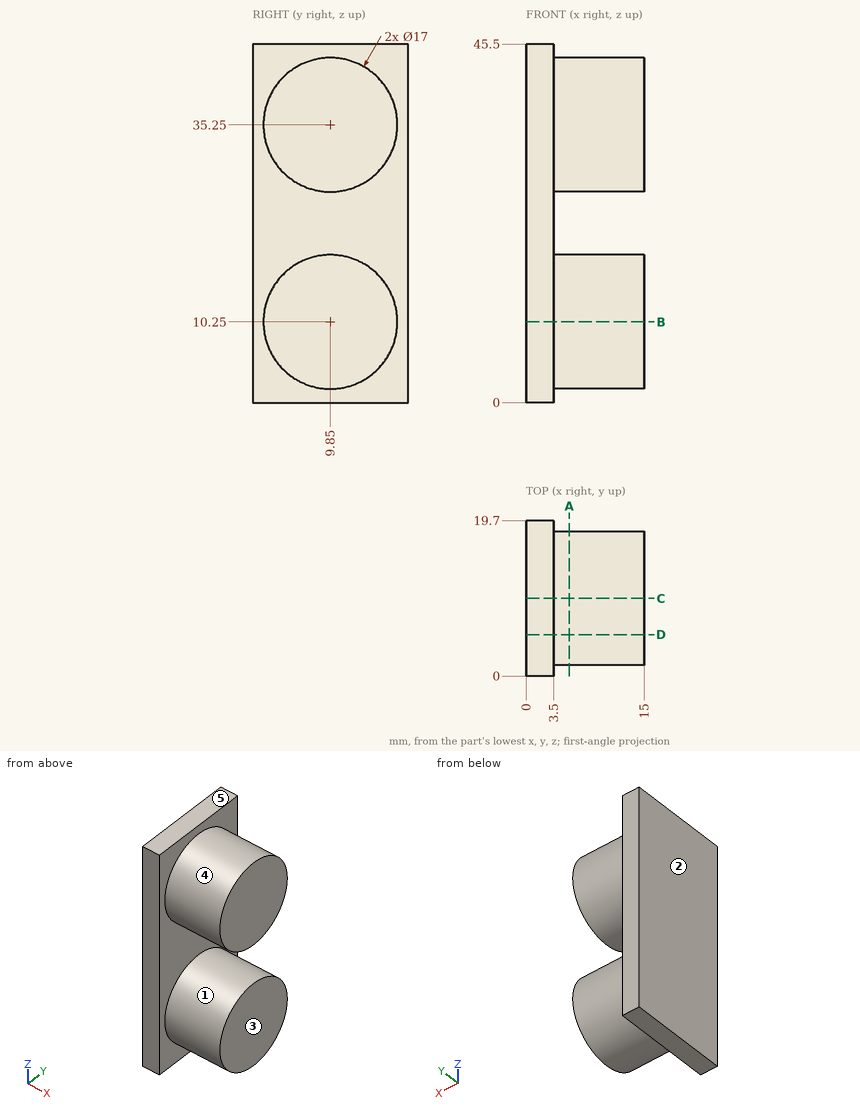
Print and shaded views of the part. All mm, measured from the part's lowest x, y and z. A direction names the side the tool comes from. Give positions to 0.01 mm unless a question says otherwise; leave off trailing zeros. Loops run counter-clockwise (first coordinate to the right, second up) from the corner with the lowest first, then second, coordinate; pieces in that order, holes last. Notation, with made-up numbers: (-33.5, 59.25) -> (-20.5, 59.25) arc R24 ccw to (-20.5, 89.25) -> close; hole circle Ø9 at (-1, -6). An arc over 180 degrees is marked (long way). One line per question, with ' | ' between items. Start each with the question number.
1) Cut at A-A (x = 5.5). Give the cut face in (y, z), plus the area to 3 significant figures.
2) Probe L1, parallel to Z at x = 6.5, y = 14.5; L2, parallel to X at y = 1.5, z = 41.5; L3, parallel to Z at x = 11.75, y = 12.5. List the from-to ranges inside material, lowest first.
3) 3-axis set-ups, long thin cutter, end or side, ignore diameter. For the marked faces 1 and 2: which of +Z, -Z, +X, -X, +Y, -Y reach the whole face in a straight line?
4) Cut at D-D (y = 5.25). Give the cut face in (x, z), plus the area to 3 significant figures.
5) Cut at C-C (y = 9.85). Give the cut face in (x, z), plus the area to 3 significant figures.
6) Cut at B-B (z = 10.25). Give the cut face in (x, y), plus the area to 3 significant figures.
7) Two-plate mould, pull along Z, no slides. Class the marked faces 3, 4 and 5: released by +Z, released by -Z, zero draft, split by the parting line, or undercut.
Return value:
1) outline: circle Ø17 at (9.85, 10.25); circle Ø17 at (9.85, 35.25) | area: 454 mm^2
2) L1: 3.13 to 17.37, 28.13 to 42.37 | L2: 0 to 3.5 | L3: 2.17 to 18.33, 27.17 to 43.33
3) face 1: +X | face 2: +Z, -Z, -X, +Y, -Y
4) outline: (0, 0) -> (3.5, 0) -> (3.5, 3.1) -> (15, 3.1) -> (15, 17.4) -> (3.5, 17.4) -> (3.5, 28.1) -> (15, 28.1) -> (15, 42.4) -> (3.5, 42.4) -> (3.5, 45.5) -> (0, 45.5) -> close | area: 488 mm^2
5) outline: (0, 0) -> (3.5, 0) -> (3.5, 1.75) -> (15, 1.75) -> (15, 18.75) -> (3.5, 18.75) -> (3.5, 26.75) -> (15, 26.75) -> (15, 43.75) -> (3.5, 43.75) -> (3.5, 45.5) -> (0, 45.5) -> close | area: 550 mm^2
6) outline: (0, 0) -> (3.5, 0) -> (3.5, 1.35) -> (15, 1.35) -> (15, 18.35) -> (3.5, 18.35) -> (3.5, 19.7) -> (0, 19.7) -> close | area: 264 mm^2
7) face 3: zero draft | face 4: undercut | face 5: released by +Z
